```python
from build123d import *

# Parameters (mm, degrees)
SKETCH2_R                        = 0.762
CHAMFER1_SIZE                    = 0.508
FILLET1_R                        = 0.254
F_10_32_TAPPED_HOLE1_D           = 4.0386
F_10_32_TAPPED_HOLE1_DEPTH       = 10.3124
F_10_32_TAPPED_HOLE1_CSINK_D     = 4.826
F_10_32_TAPPED_HOLE1_CSINK_ANGLE = 90
F_10_32_TAPPED_HOLE1_TIP         = 1.213317848


with BuildPart() as part:
    # Sketch1 → Revolve1 (revolve)
    with BuildSketch(Plane.XY, mode=Mode.PRIVATE) as revolve1_sk:
        Polygon((12.7, 0), (6.35, 0), (6.35, -6.35), (0, -6.35), (0, 17.78), (1.5875, 17.78), (12.7, 6.6675), align=None)
    revolve(revolve1_sk.sketch.rotate(Axis((0, 35.289344262, 0), (0, -1, 0)), 90), axis=Axis((0, 35.289344262, 0), (0, -1, 0)))  # turned: the seam where the file's is

    # Sketch2 → Cut-Revolve1 (revolve, cut)
    with BuildSketch(Plane.XY, mode=Mode.PRIVATE) as cut_revolve1_sk:
        with Locations((6.858, -0.508)):
            Circle(SKETCH2_R)
    revolve(cut_revolve1_sk.sketch.rotate(Axis((0, 0, 0), (0, -1, 0)), 90), axis=Axis((0, 0, 0), (0, -1, 0)), mode=Mode.SUBTRACT)  # turned: the seam where the file's is

    # Chamfer1
    chamfer1_edges = [part.edges().sort_by_distance(p)[0] for p in [
        (0, -6.35, -6.35),
    ]]
    chamfer(chamfer1_edges, length=CHAMFER1_SIZE)

    # Fillet1
    fillet1_edges = [part.edges().sort_by_distance(p)[0] for p in [
        (0, 0, -12.7),
    ]]
    fillet(fillet1_edges, radius=FILLET1_R)

    # 10-32 Tapped Hole1
    with Locations(Plane.XZ.offset(6.35)):
        with Locations((0, 0)):
            CounterSinkHole(F_10_32_TAPPED_HOLE1_D / 2, F_10_32_TAPPED_HOLE1_CSINK_D / 2, depth=F_10_32_TAPPED_HOLE1_DEPTH, counter_sink_angle=F_10_32_TAPPED_HOLE1_CSINK_ANGLE)
            with Locations((0, 0, -(F_10_32_TAPPED_HOLE1_DEPTH + F_10_32_TAPPED_HOLE1_TIP / 2))):  # 118° drill point
                Cone(0, F_10_32_TAPPED_HOLE1_D / 2, F_10_32_TAPPED_HOLE1_TIP, mode=Mode.SUBTRACT)


solid = part.part
```
Design review of the part built by this model. Coordinates are the model's own, in mm. A direction names the side the tool comes from. Coordinates: 2 decimals unless noted, no trailing zeros. Write each loop counter-clockwise with the first axis right and the second up, starting at its lowest first coordinate (ties: lowest second). Pieces come first, ordered by that corner, then holes. Notation, with made-up numbers: M 42,32 L 53,32 A10 ccw 53,48 Z; hole C 52,2 d2. An arc over 180 degrees is marked long. Answer as a JSON object with one key per item and string values.
Item 1: Draft analysis for pull direction X (two halves, no side actions). For faces 1 (the cylindrical face through (7.7, 3.4, -10.1)), 2 (the cylindrical face through (-1.926, -0.928, 0.607)), 3 (the conical face through (-0.076, 4.965, -0.342)), 4 (the flat face through (0, 17.78, 0)), state which applies: pulls with the +X half, pulls with the -X half, needs draft (parallel to the pull), parting line crosses it, or undercut.
Outcome:
{"face 1": "parting line crosses it", "face 2": "undercut", "face 3": "undercut", "face 4": "needs draft"}
Item 2: Wall thickness on probe 1 along X at (y, z) = (-3.25, 0); probe 2 along X at (y, z) = (3, 0); probe 3 along Y at (x, z) = (-8.5, 4.5): over which ranges is each line inside the solid? List them lowest first.
Outcome:
{"probe 1": "-6.35 to -2.02, 2.02 to 6.35", "probe 2": "-12.7 to -2.02, 2.02 to 12.7", "probe 3": "0 to 9.75"}
Item 3: Insertion check: pin 1 Ø5 at (y, z) = (12.5, -9) entering from -X; pin 2 Ø1 at (x, z) = (-4, -0.5) entering from +Y; pin 3 Ø3.5 at (x, z) = (0, 0) entering from -Y. Each pin has a flat end and moves straight along its axis. Give the tip position at first contact, or say it passes through.
Outcome:
{"pin 1": "x = -4.74", "pin 2": "y = 15.84", "pin 3": "y = 4.12"}
Item 4: Machinability: for faces 5 (the conical face through (-1.057, 15.85, 3.355)), 6 (the cylindrical face through (3.86, -3.49, -5.04)), which of the approach directions +Z, -Z, +X, -X, +Y, -Y give a long, thin tool a straight path to every point of the face, cutting with its end or side? Answer none if there is none.
Outcome:
{"face 5": "+Y", "face 6": "-Y"}
Item 5: Add section A-A, the plane y = 0.75. Give the boundary of the cut face in (x, z), and give its area (3 significant figures).
Outcome:
{"outline": "C 0,0 d25.4; hole C 0,0 d4.04", "area": "494 mm²"}
Item 6: Add section B-B, the plane y = 13. Give the boundary of the cut face in (x, z) (1 decimal).
Outcome:
{"outline": "C 0,0 d12.7"}
Item 7: Add section C-C, the plane y = -2.75. Give the boundary of the cut face in (x, z), and give its area (3 significant figures).
Outcome:
{"outline": "C 0,0 d12.7; hole C 0,0 d4.04", "area": "114 mm²"}
Item 8: Add section D-D, the plane y = 9.25. Give the boundary of the cut face in (x, z) (1 decimal).
Outcome:
{"outline": "C 0,0 d20.2"}
